Source: three-view drawing plus pictorial views. Frame: mm from the lowest corner of the part. A direction names the side the tool comes from. Give positions to 0.01 mm unless a question says otherwise; leave off trailing zeros. Write each loop counter-clockwise with the first axis right and the second up, starting at its lowest first coordinate (ties: lowest second). Pieces come first, ordered by that corner, then holes.
Q1. Reachability of the marked faces 1 and 2 from +Z, -Z, +X, -X, +Y, -Y: full face, straight path, thin tool, end or side. Return the list, or none.
Q2. Cut plane D-D on z = 12.5. Return the cut outline in (x, y).
Q3. Line query: L1, parallel to X at y = 1.2, z = 8.5; L2, parallel to Z at x = 21, y = 2.5; L3, parallel to X at y = 1.15, z = 12.5. Output: solid intervals per line, ascending.
Q4. Draft query along X for the marked faces 3, 4 and 5. Return one class per face: pulls with the +X half, pulls with the -X half, needs draft (parallel to the pull), parting line crosses it, or undercut.
Q5. Cut plane C-C on y = 0.3. Return the cut outline in (x, z).
Q6. Cut plane A-A on z = 8.5. Return the cut outline in (x, y).
Q7. Cut plane B-B on x = 3.5. Return the cut outline in (y, z).
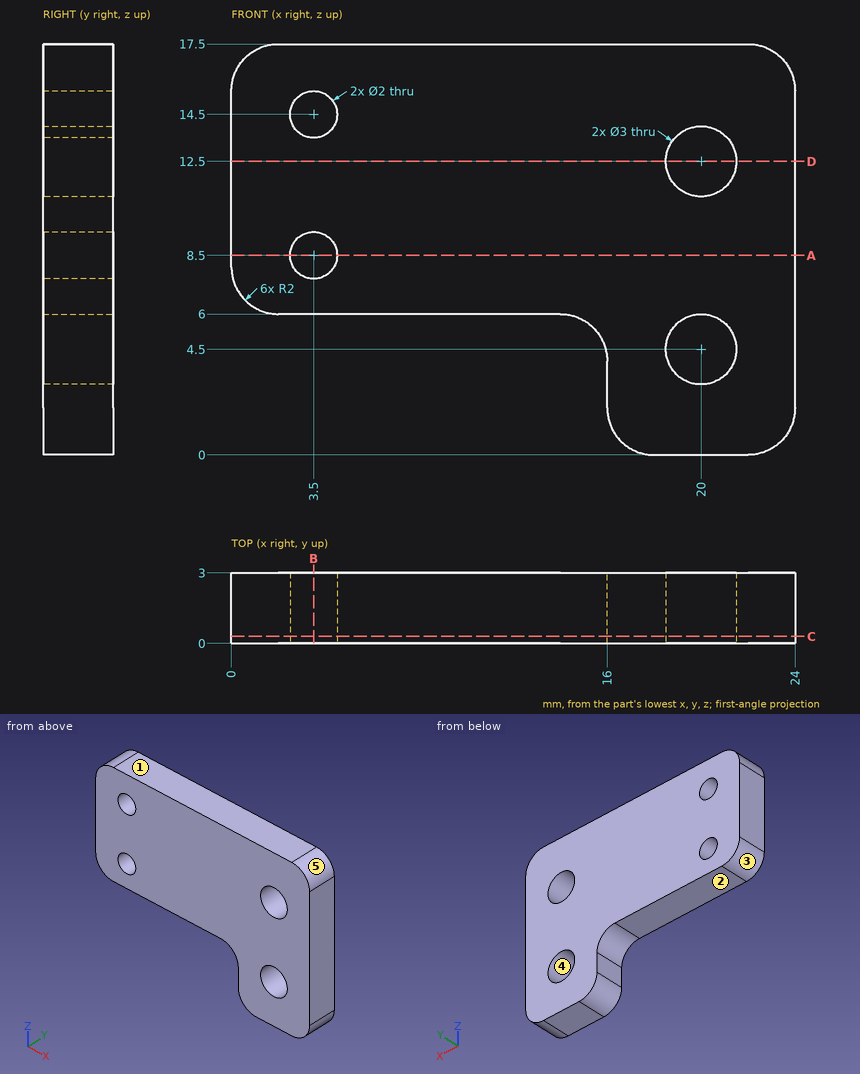
Data:
1. face 1: +Z, +X, -X, +Y, -Y
1. face 2: -Z, -X, +Y, -Y
2. outline: (0, 0) - (18.5, 0) - (18.5, 3) - (0, 3) - close; (21.5, 0) - (24, 0) - (24, 3) - (21.5, 3) - close
3. L1: x = 0 to 2.5, 4.5 to 24
3. L2: z = 0 to 3.38, 5.62 to 11.38, 13.62 to 17.5
3. L3: x = 0 to 18.5, 21.5 to 24
4. face 3: pulls with the -X half
4. face 4: undercut
4. face 5: pulls with the +X half
5. outline: (0, 8) arc R2 ccw to (2, 6) - (14, 6) arc R2 cw to (16, 4) - (16, 2) arc R2 ccw to (18, 0) - (22, 0) arc R2 ccw to (24, 2) - (24, 15.5) arc R2 ccw to (22, 17.5) - (2, 17.5) arc R2 ccw to (0, 15.5) - close; hole circle Ø2 at (3.5, 8.5); hole circle Ø2 at (3.5, 14.5); hole circle Ø3 at (20, 4.5); hole circle Ø3 at (20, 12.5)
6. outline: (0, 0) - (2.5, 0) - (2.5, 3) - (0, 3) - close; (4.5, 0) - (24, 0) - (24, 3) - (4.5, 3) - close
7. outline: (0, 6) - (3, 6) - (3, 7.5) - (0, 7.5) - close; (0, 9.5) - (3, 9.5) - (3, 13.5) - (0, 13.5) - close; (0, 15.5) - (3, 15.5) - (3, 17.5) - (0, 17.5) - close
